Job drawing, mm, ordinate dimensions from the low corner. One solid piece. A direction names the side the tool comes from. Give positions to 0.01 mm unless a question says otherwise; leave off trailing zeros. Loops run counter-clockwise (first coordinate to the right, second up) from the corner with the lowest first, then second, coordinate; pieces in that order, holes last. Notation, with made-up numbers: (61.25, 0) - (116.25, 0) arc R28 cw to (116.25, 35) - close; hole circle Ø6 at (77, 78.25). An arc over 180 degrees is marked (long way). Use a Markdown table: item, result.
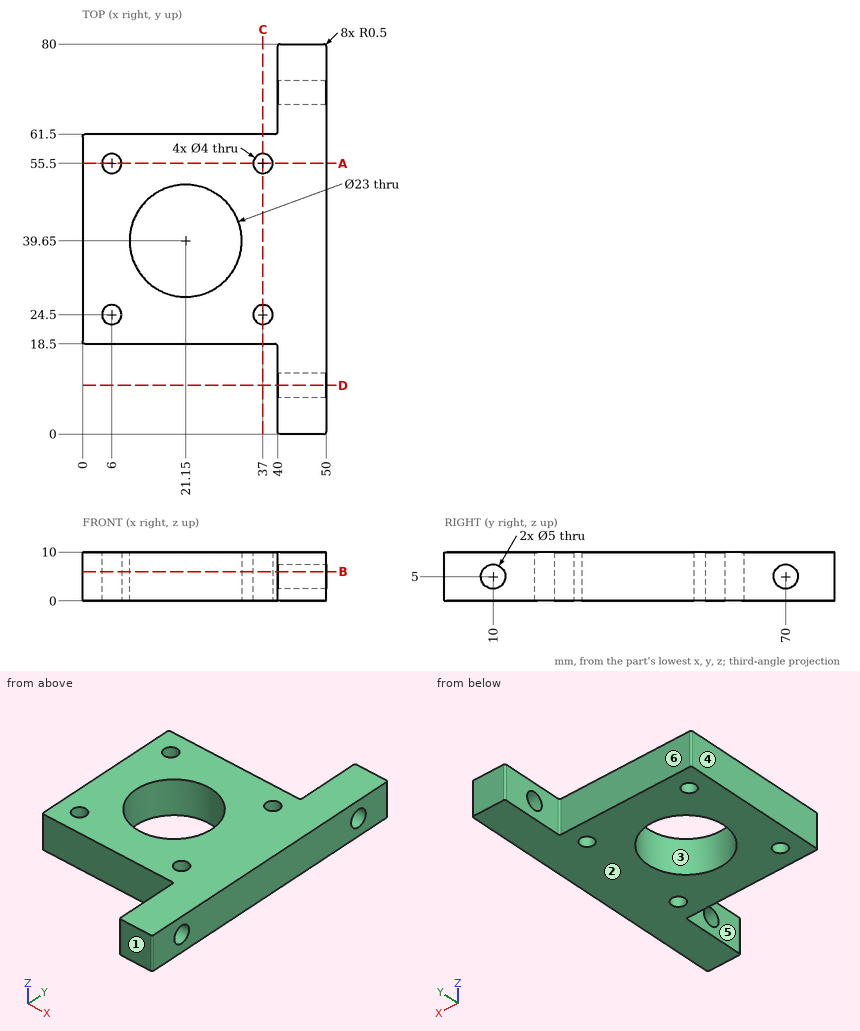
(1) Mould opens along Y. For the marked faces 1, 2 and 3 say: pulls with the +Y half, pulls with the -Y half, needs draft (parallel to the pull), parting line crosses it, or undercut.
Computed:
| item | result |
|---|---|
| face 1 | pulls with the -Y half |
| face 2 | needs draft |
| face 3 | undercut |
(2) Slice it at B-B, the plane z = 6. Count the separate pieces of the cut face and the enclosed holes in it, plus the area to 3 significant figures.
Computed:
| item | result |
|---|---|
| separate pieces | 3 |
| enclosed holes | 5 |
| area | 1,960 mm² |
(3) Drill centre lines: probe 1 along Y at (x, z) = (6, 3); probe 2 along X at (y, z) = (24.5, 4); probe 3 along Y at (x, z) = (21.15, 8). Where is each one in solid material? Low to high. Write a range as [from, to].
Computed:
| item | result |
|---|---|
| probe 1 | [18.5, 22.5], [26.5, 53.5], [57.5, 61.5] |
| probe 2 | [0, 4], [8, 35], [39, 50] |
| probe 3 | [18.5, 28.15], [51.15, 61.5] |
(4) Slice it at D-D, the plane y = 10. Write the cut outline in (x, z), plus the area to 3 significant figures.
Computed:
| item | result |
|---|---|
| outline | (40, 0) - (50, 0) - (50, 2.5) - (40, 2.5) - close; (40, 7.5) - (50, 7.5) - (50, 10) - (40, 10) - close |
| area | 50.0 mm² |
(5) Slice it at C-C, the plane x = 37. Write the cut outline in (y, z), plus the area to 3 significant figures.
Computed:
| item | result |
|---|---|
| outline | (18.5, 0) - (22.5, 0) - (22.5, 10) - (18.5, 10) - close; (26.5, 0) - (53.5, 0) - (53.5, 10) - (26.5, 10) - close; (57.5, 0) - (61.5, 0) - (61.5, 10) - (57.5, 10) - close |
| area | 350 mm² |
(6) 3-axis set-ups, long thin cutter, end or side, ignore diameter. For the marked faces 4, 5 and 6: which of +Z, -Z, +X, -X, +Y, -Y reach the whole face in a straight line?
Computed:
| item | result |
|---|---|
| face 4 | +Z, -Z, -X, +Y, -Y |
| face 5 | +Z, -Z, -X, -Y |
| face 6 | +Z, -Z, -X, +Y |
(7) Pin check, flat tips, straight feed: P1, Ø5, axis at x = 11.5, z = 4, coming from the +Y side; P2, Ø1.5, axis at x = 26.5, z = 3, coming from the -Y side. Stop position of each tip, or through.
Computed:
| item | result |
|---|---|
| P1 | y = 61.5 |
| P2 | y = 18.5 |
(8) Slice it at A-A, the plane y = 55.5. Write the cut outline in (x, z).
Computed:
| item | result |
|---|---|
| outline | (0, 0) - (4, 0) - (4, 10) - (0, 10) - close; (8, 0) - (35, 0) - (35, 10) - (8, 10) - close; (39, 0) - (50, 0) - (50, 10) - (39, 10) - close |
